Autodesk Inventor part; units mm, degrees
ref_plane "YZ Plane" through (0, 0, 0) normal (1, 0, 0) x (0, 1, 0)
ref_plane "XZ Plane" through (0, 0, 0) normal (0, 1, 0) x (-1, 0, 0)
ref_plane "XY Plane" through (0, 0, 0) normal (0, 0, 1) x (1, 0, 0)
sketch "Sketch3" plane through (0, 0, 0) normal (0, 0, 1) x (1, 0, 0)
  line L0 (0, 0) -> (0, 4.572)
  line L1 (0, 4.572) -> (4.2333, 5.2324)
  line L2 (0, 0) -> (21.1667, 0)
  line L3 (4.2333, 5.2324) -> (4.2333, 4.572)
  line L4 (4.2333, 4.572) -> (8.4667, 5.2324)
  line L5 (8.4667, 5.2324) -> (8.4667, 4.572)
  line L6 (8.4667, 4.572) -> (12.7, 5.2324)
  line L7 (12.7, 5.2324) -> (12.7, 4.572)
  line L8 (12.7, 4.572) -> (16.9333, 5.2324)
  line L9 (16.9333, 5.2324) -> (16.9333, 4.572)
  line L10 (16.9333, 4.572) -> (21.1667, 5.2324)
  line L11 (21.1667, 5.2324) -> (21.1667, 0)
  line L12 (21.1667, 0) -> (24.3417, 0)
  line L13 (24.3417, 0) -> (24.3417, 6.35)
  line L14 (24.3417, 6.35) -> (21.1667, 6.35)
  line L15 (21.1667, 6.35) -> (21.1667, 0)
  dimension "d4" = 4.572
  dimension "d6" = 5.2324
  dimension "d7" = 4.2333
  dimension "d8" = 3.175
  dimension "d9" = 6.35
revolve "Revolution1" add sketch "Sketch3" angle 360 about axis through (0, 0, 0) along (1, 0, 0)
sketch "Sketch4" plane through (0, 0, 0) normal (-1, 0, 0) x (0, 0, 1)
  circle A0 centre (0, 0) radius 3.6322
  dimension "d11" = 7.2644
sketch "Sketch5" plane through (24.3417, 0, 0) normal (1, 0, 0) x (0, 0, -1)
  circle A0 centre (0, 0) radius 1.5875
  dimension "d15" = 3.175
loft "Loft1" cut profiles "Sketch4", "Sketch5"
fillet "Fillet2" radius 0.7937 1 edges at (0, 0, -3.6322)
sketch "Sketch6" plane through (24.3417, 0, 0) normal (1, 0, 0) x (0, 0, -1)
  circle A0 centre (0, 0) radius 6.35
  line L0 (-10.16, 10.16) -> (10.16, 10.16) construction
  line L1 (10.16, 10.16) -> (10.16, -10.16) construction
  line L2 (10.16, -10.16) -> (-10.16, -10.16) construction
  line L3 (-10.16, -10.16) -> (-10.16, 10.16) construction
  line L4 (-10.16, 10.16) -> (10.16, -10.16) construction
  line L5 (-10.16, -10.16) -> (10.16, 10.16) construction
  circle A1 centre (-10.16, 10.16) radius 1.1
  circle A2 centre (10.16, 10.16) radius 1.1
  circle A3 centre (10.16, -10.16) radius 1.1
  circle A4 centre (-10.16, -10.16) radius 1.1
  circle A5 centre (-10.16, 10.16) radius 2.37
  circle A6 centre (10.16, 10.16) radius 2.37
  circle A7 centre (10.16, -10.16) radius 2.37
  circle A8 centre (-10.16, -10.16) radius 2.37
  arc A9 (-6.35, 0) -> (-11.2499, 8.0555) centre (-15.4216, 0) ccw
  arc A10 (-8.0555, 11.2499) -> (0, 6.35) centre (0, 15.4216) ccw
  arc A11 (0, -6.35) -> (-8.0555, -11.2499) centre (0, -15.4216) ccw
  arc A12 (-11.2499, -8.0555) -> (-6.35, 0) centre (-15.4216, 0) ccw
  arc A13 (6.35, 0) -> (11.2499, -8.0555) centre (15.4216, 0) ccw
  arc A14 (8.0555, -11.2499) -> (0, -6.35) centre (0, -15.4216) ccw
  arc A15 (0, 6.35) -> (8.0555, 11.2499) centre (0, 15.4216) ccw
  arc A16 (11.2499, 8.0555) -> (6.35, 0) centre (15.4216, 0) ccw
  point P0 (0, 0)
  point P1 (6.35, 0)
  point P2 (6.35, 0)
  point P3 (6.35, 0)
  point P4 (8.0555, 11.2499)
  point P5 (0, 6.35)
  point P6 (0, 6.35)
  point P7 (0, -6.35)
  point P8 (0, -6.35)
  point P9 (0, -6.35)
  point P10 (8.0555, -11.2499)
  point P11 (11.2499, -8.0555)
  point P12 (-6.35, 0)
  point P13 (-6.35, 0)
  point P14 (-11.2499, -8.0555)
  point P15 (-8.0555, -11.2499)
  dimension "d21" = 20.32
  dimension "d22" = 2.2
  dimension "d23" = 1.27
  dimension "d26" = 360
extrude "Extrusion3" add sketch "Sketch6" against normal blind 3.175 contours A13 A7 A14 A0 | A0 A15 A6 A16 | A0 A9 A5 A10 | A11 A8 A12 A0 | A7 | A6 | A5 | A8
fillet "Fillet3" radius 0.7937 1 edges at (24.3417, 0, -1.5875)
properties part number "NozzleAdapter"
Model file for the job. Use its own axes, mm. A direction names the side the tool comes from. Give positions to 0.01 mm unless a question says otherwise; leave off trailing zeros. Write each loop counter-clockwise with the first axis right and the second up, starting at its lowest first coordinate (ties: lowest second). Pieces come first, ordered by that corner, then holes. Notation, with made-up numbers: (75.25, 36.25) -> (127.25, 36.25) arc R7 ccw to (127.25, 43.25) -> close; hole circle Ø8 at (75, 53). An arc over 180 degrees is marked (long way). Use CSV: the item, a comma, the result in double quotes. Start each with the question number.
1) Cut at A-A on z = -10.16. List the corners of the cut face in (x, y).
2) Cut at D-D on z = -7.5. List the corners of the cut face in (x, y), plus the area to 3 significant figures.
3) Drill centre lines: L1, parallel to Y at x = 23.35, z = -10.16; L2, parallel to Y at x = 11.25, z = 0.5; L3, parallel to X at y = 6.25, z = 4. Where is each one in solid material? Low to high.
4) Two-plate mould, pull along Y, no slides. Class faces 1 (the cylindrical face through (22.776, 4.655, 7.635)), 2 (the flat face through (12.7, 0, -5)), 3 (the cylindrical face through (22.776, 7.635, -4.655)): released by +Y, released by -Y, zero draft, split by the parting line, or undercut.
5) Tool access for faces 4 (the cylindrical face through (22.776, -7.707, -4.774)), 5 (the cylindrical face through (22.776, -4.655, -7.635)), 6 (the flat face through (8.467, 0, -5)): list every direction of +Z, -Z, +X, -X, +Y, -Y with a clear straight run to the whole face (end or side of a thin tool).
6) Cut at C-C on x = 22. List the corners of the cut face in (y, z), plus the area to 3 significant figures.
7) Pin check, flat tips, straight feed: P1, Ø12, axis at x = 10, y = 1, coming from the +Z side; P2, Ø3, axis at x = 16.5, y = -4.5, coming from the -Z side; P3, Ø1, axis at y = -2.5, z = 6, coming from the -X side. Stop position of each tip, or through.
Final values:
1,outline,"(21.17, -12.53) -> (24.34, -12.53) -> (24.34, -11.26) -> (21.17, -11.26) -> close; (21.17, -9.06) -> (24.34, -9.06) -> (24.34, -7.39) -> (21.17, -7.39) -> close; (21.17, 7.39) -> (24.34, 7.39) -> (24.34, 9.06) -> (21.17, 9.06) -> close; (21.17, 11.26) -> (24.34, 11.26) -> (24.34, 12.53) -> (21.17, 12.53) -> close"
2,outline,"(21.17, -10.32) -> (24.34, -10.32) -> (24.34, -4.42) -> (21.17, -4.42) -> close; (21.17, 4.42) -> (24.34, 4.42) -> (24.34, 10.32) -> (21.17, 10.32) -> close"
2,area,"37.4 mm2"
3,L1,"y = -12.53 to -11.26, -9.06 to -7.39, 7.39 to 9.06, 11.26 to 12.53"
3,L2,"y = -4.98 to -2.64, 2.64 to 4.98"
3,L3,"x = 21.17 to 24.34"
4,face 1,"undercut"
4,face 2,"zero draft"
4,face 3,"released by +Y"
5,face 4,"+X, -X, -Y"
5,face 5,"-Z, +X, -X"
5,face 6,"none"
6,outline,"(-11.25, -8.06) arc R2.37 ccw (long way) to (-8.06, -11.25) arc R9.07 cw to (0, -6.35) arc R9.07 cw to (8.06, -11.25) arc R2.37 ccw (long way) to (11.25, -8.06) arc R9.07 cw to (6.35, 0) arc R9.07 cw to (11.25, 8.06) arc R2.37 ccw (long way) to (8.06, 11.25) arc R9.07 cw to (0, 6.35) arc R9.07 cw to (-8.06, 11.25) arc R2.37 ccw (long way) to (-11.25, 8.06) arc R9.07 cw to (-6.35, 0) arc R9.07 cw to start; hole circle Ø2.2 at (-10.16, -10.16); hole circle Ø2.2 at (-10.16, 10.16); hole circle Ø3.57 at (0, 0); hole circle Ø2.2 at (10.16, -10.16); hole circle Ø2.2 at (10.16, 10.16)"
6,area,"284 mm2"
7,P1,"stops at z = 5.23"
7,P2,"stops at z = -4.24"
7,P3,"stops at x = 21.17"
